from build123d import *

# Parameters (mm, degrees)
SKETCH1_W           = 500
SKETCH1_H           = 500
SKETCH1_W_2         = 496
SKETCH1_H_2         = 496
EXTRUDE_THIN1_DEPTH = 500
SKETCH2_W           = 500
SKETCH2_H           = 500
SKETCH2_W_2         = 496
SKETCH2_H_2         = 496
EXTRUDE_THIN2_DEPTH = 250
CUT_EXTRUDE1_REACH  = 752
SKETCH3_W           = 496
SKETCH3_H           = 496


with BuildPart() as part:
    # Sketch1 → Extrude-Thin1 (new body, symmetric)
    with BuildSketch(Plane(origin=(0, 0, 0), x_dir=(0, 0, -1), z_dir=(1, 0, 0))):
        Rectangle(SKETCH1_W, SKETCH1_H)
        Rectangle(SKETCH1_W_2, SKETCH1_H_2, mode=Mode.SUBTRACT)
    extrude(amount=EXTRUDE_THIN1_DEPTH, both=True)

    # Sketch2 → Extrude-Thin2 (add)
    with BuildSketch(Plane(origin=(0, -250, 250), x_dir=(1, 0, 0), z_dir=(0, 0, -1))):
        with Locations((0, -250)):
            Rectangle(SKETCH2_W, SKETCH2_H)
        with Locations((0, -250)):
            Rectangle(SKETCH2_W_2, SKETCH2_H_2, mode=Mode.SUBTRACT)
    extrude(amount=-EXTRUDE_THIN2_DEPTH)

    # Sketch3 → Cut-Extrude1 (cut, up to next)
    with BuildSketch(Plane(origin=(0, -750, 500), x_dir=(1, 0, 0), z_dir=(0, 0, -1)), mode=Mode.PRIVATE) as cut_extrude1_sk1:
        with Locations((0, -750)):
            Rectangle(SKETCH3_W, SKETCH3_H)
    cut_extrude1_tool1 = extrude(cut_extrude1_sk1.sketch, amount=CUT_EXTRUDE1_REACH, mode=Mode.PRIVATE) & part.part
    add(cut_extrude1_tool1.solids().sort_by_distance((0, 0, 500))[0], mode=Mode.SUBTRACT)


solid = part.part
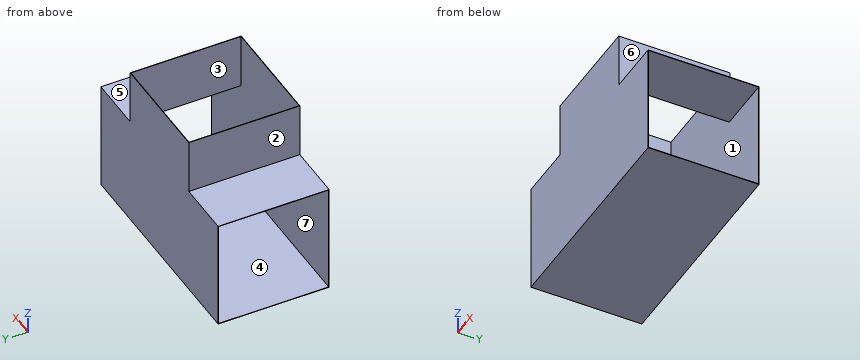
Build history of the part. All positions in model axes, mm. Face numbers are marked on the shaded views. A direction names the side the tool comes from. Coordinates: 2 decimals unless noted, no trailing zeros. Write each loop counter-clockwise with the first axis right and the second up, starting at its lowest first coordinate (ties: lowest second). Pieces come first, ordered by that corner, then holes. Notation, with made-up numbers: (-15, 42) -> (20, 42) arc R22 ccw to (20, 55) -> close; hole circle Ø2 at (22.25, -32). An arc over 180 degrees is marked (long way). Use CSV: the item, a comma, the result in double quotes. Start each with the question number.
Q1. Pull direction Z, two halves, no side cores. Call the marked faces 5, 6 and 7: released by +Z, released by -Z, zero draft, split by the parting line, or undercut.
Q2. 3-axis set-ups, long thin cutter, end or side, ignore diameter. For the marked faces 1, 2, 3 and 4: which of +Z, -Z, +X, -X, +Y, -Y reach the whole face in a straight line?
Q3. Cut at B-B, the plane x = -309. List the corners of the cut face in (y, z), then the cut area to 3 significant figures.
Q4. Cut at C-C, the plane y = 195. List the corners of the cut face in (x, z), then the cut area to 3 significant figures.
Q5. Flat gauge pins, fed straight in: pin 1 Ø8 at (x, y) = (149.5, -174) entering from +Z; pin 2 Ø1 at (y, z) = (-54, 314) entering from +X; pin 3 Ø2 at (x, y) = (295, -118) entering from +Z. Where does each tip first touch, or does it go through?
Q6. Drill centre line: probe 1 along Z at (x, y) = (-254.5, 101). Where is it in solid material? Low to high.
Q7. Cut at A-A, the plane z = -147. List the corners of the cut face in (x, y), then the cut area to 3 significant figures.
Checked values:
1,face 5,"released by +Z"
1,face 6,"zero draft"
1,face 7,"undercut"
2,face 1,"none"
2,face 2,"+Z, -X, +Y, -Y"
2,face 3,"+Z"
2,face 4,"+X, -X"
3,outline,"(-250, -250) -> (250, -250) -> (250, 250) -> (-250, 250) -> close; hole (-248, -248) -> (248, -248) -> (248, 248) -> (-248, 248) -> close"
3,area,"3,980 mm²"
4,outline,"(-500, -250) -> (500, -250) -> (500, -248) -> (-500, -248) -> close; (-500, 248) -> (-248, 248) -> (-248, 500) -> (-250, 500) -> (-250, 250) -> (-500, 250) -> close; (248, 248) -> (500, 248) -> (500, 250) -> (250, 250) -> (250, 500) -> (248, 500) -> close"
4,area,"4,010 mm²"
5,pin 1,"stops at z = -248"
5,pin 2,"stops at x = 250"
5,pin 3,"stops at z = 250"
6,probe 1,"z = -250 to -248, 248 to 250"
7,outline,"(-500, -250) -> (500, -250) -> (500, -248) -> (-500, -248) -> close; (-500, 248) -> (500, 248) -> (500, 250) -> (-500, 250) -> close"
7,area,"4,000 mm²"
